Source: CAD feature listing. Evaluate the final solid. Frame: model axes, mm. Give positions to 0.01 mm unless a question says otherwise; leave off trailing zeros. Write each loop counter-clockwise with the first axis right and the second up, starting at its lowest first coordinate (ties: lowest second). Pieces come first, ordered by that corner, then holes. Notation, with made-up numbers: (26, 63.5) -> (75, 63.5) arc R27 ccw to (75, 102.5) -> close; hole circle Ø10 at (52, 27.5). An arc over 180 degrees is marked (long way). Write item = value, one per line.
from build123d import *

# Parameters (mm, degrees)
F0_W     = 20
F0_H     = 20
F1_DEPTH = 2
F3_D     = 2.5
F4_R     = 1.5
F5_DEPTH = 25


with BuildPart() as f1:
    # F0 (on Top) → F1 (new body)
    with BuildSketch(Plane.XY):
        Rectangle(F0_W, F0_H)
    extrude(amount=-F1_DEPTH)

    # F3 (through all)
    with Locations(Plane.XY):
        with Locations((-7, 7), (7, 7), (-7, -7), (7, -7)):
            Hole(F3_D / 2)

    # F4 (on face) → F5 (cut)
    with BuildSketch(Plane.XY):
        Circle(F4_R)
    extrude(amount=-F5_DEPTH, mode=Mode.SUBTRACT)


solid = f1.part
1) Draft query along Y for faces 1 (the flat face through (0, -10, -1)), 2 (the flat face through (0, 10, -1)), 3 (the cylindrical face through (-6.01, -7.76, -1.01)). Return one class per face: pulls with the +Y half, pulls with the -Y half, needs draft (parallel to the pull), parting line crosses it, or undercut.
Computed:
face_1 = pulls with the -Y half
face_2 = pulls with the +Y half
face_3 = undercut
2) Cut plane A-A (x = 0). Return the cut outline in (y, z).
Computed:
outline = (-10, -2) -> (-1.5, -2) -> (-1.5, 0) -> (-10, 0) -> close; (1.5, -2) -> (10, -2) -> (10, 0) -> (1.5, 0) -> close
3) Material intervals for L1, parallel to Y at x = 7, z = -0.85; L2, parallel to Y at x = 0, z = -1.3; L3, parallel to X at y = 7.5, z = -1.75, sorted ascending.
Computed:
L1 = -10 to -8.25, -5.75 to 5.75, 8.25 to 10
L2 = -10 to -1.5, 1.5 to 10
L3 = -10 to -8.15, -5.85 to 5.85, 8.15 to 10
4) Cut plane B-B (y = 7). Return the cut outline in (x, z), then the cut area to 3 significant figures.
Computed:
outline = (-10, -2) -> (-8.25, -2) -> (-8.25, 0) -> (-10, 0) -> close; (-5.75, -2) -> (5.75, -2) -> (5.75, 0) -> (-5.75, 0) -> close; (8.25, -2) -> (10, -2) -> (10, 0) -> (8.25, 0) -> close
area = 30.0 mm²
5) Contact query for a flat-ended pin moving along its axis: pin 1 (2 mm diameter, centred on x = -7, y = -7, fed in from +Z). Output: stop coordinate, or through.
Computed:
pin_1 = through
6) Cut plane C-C (z = -1.3). Return the cut outline in (x, y), then the cut area to 3 significant figures.
Computed:
outline = (-10, -10) -> (10, -10) -> (10, 10) -> (-10, 10) -> close; hole circle Ø2.5 at (-7, -7); hole circle Ø2.5 at (-7, 7); hole circle Ø3 at (0, 0); hole circle Ø2.5 at (7, -7); hole circle Ø2.5 at (7, 7)
area = 373 mm²
